from build123d import *

# Parameters (mm, degrees)
SKETCH1_W                   = 32.5
SKETCH1_H                   = 4.2
BASEFORM_DEPTH              = 7
SKETCH2_R                   = 0.75
HUMERUSAXLEHOLE1_DEPTH      = 2
HUMERUSAXLELOCK_DEPTH       = 1
SKETCH6_R                   = 1.5
AXLEEXTENSION_DEPTH         = 6
SKETCH7_R                   = 0.6
SCREWHOLES_DEPTH            = 54.273445543
SCREWHOLES_DEPTH_BACK       = 54.273445543
SKETCH8_W                   = 2.5
SKETCH8_H                   = 2.5
HUMERUSTUBEHOLDERBASE_DEPTH = 4.2
SKETCH13_W                  = 1.5
SKETCH13_H                  = 1.5
TUBECLIPENTRANCE_DEPTH      = 2
SKETCH14_W                  = 1.5
SKETCH14_H                  = 1.5
CABLECLIPLOCKSLOT_DEPTH     = 0.7
SKETCH15_W                  = 1.5
SKETCH15_H                  = 0.2
TUBECLIPLOCKCLEARANCE_DEPTH = 2
SKETCH12_R                  = 0.75
HUMERUSAXLEHOLE2_DEPTH      = 54.818584249


with BuildPart() as part:
    # Sketch1 → BaseForm (new body)
    with BuildSketch(Plane.XY):
        Polygon((0, -2.584500111), (0, 2.584500111), (3.25, 4.1), (39.25, 4.1), (42.5, 2.584500111), (42.5, -2.584500111), (39.25, -4.1), (3.25, -4.1), align=None)
        with Locations((21.25, 0)):
            Rectangle(SKETCH1_W, SKETCH1_H, mode=Mode.SUBTRACT)
    extrude(amount=BASEFORM_DEPTH)

    # Sketch2 → HumerusAxleHole1 (cut)
    with BuildSketch(Plane(origin=(0, 4.1, 0), x_dir=(1, 0, 0), z_dir=(0, 1, 0))):
        with Locations(Location((21.25, -3.5, 0), (0, 0, 270))):
            Circle(SKETCH2_R)
    extrude(amount=-HUMERUSAXLEHOLE1_DEPTH, mode=Mode.SUBTRACT)

    # Sketch2_4 → HumerusAxleLock (cut)
    with BuildSketch(Plane(origin=(0, 4.1, 0), x_dir=(1, 0, 0), z_dir=(0, 1, 0))):
        with BuildLine():
            ThreePointArc((20.65, -3.05), (21.25, -2.75), (21.85, -3.05))
            Line((21.85, -3.05), (21.85, -1.5))
            Line((21.85, -1.5), (20.65, -1.5))
            Line((20.65, -1.5), (20.65, -3.05))
        make_face()
        with BuildLine():
            Line((21.85, -5.5), (21.85, -3.95))
            ThreePointArc((21.85, -3.95), (21.25, -4.25), (20.65, -3.95))
            Line((20.65, -3.95), (20.65, -5.5))
            Line((20.65, -5.5), (21.85, -5.5))
        make_face()
    extrude(amount=-HUMERUSAXLELOCK_DEPTH, mode=Mode.SUBTRACT)

    # Sketch5 → Axle (revolve)
    with BuildSketch(Plane.XY.offset(3.5), mode=Mode.PRIVATE) as axle_sk:
        Polygon((53, 0), (53, 1.5), (46.5, 1.5), (44, 2.584500111), (42.5, 2.584500111), (42.5, 0), align=None)
    axle = revolve(axle_sk.sketch.rotate(Axis((42.5, 0, 3.5), (1, 0, 0)), 90), axis=Axis((42.5, 0, 3.5), (1, 0, 0)))

    # Axle2: Axle across plane
    add(axle.mirror(Plane.ZY.offset(-21.25)))

    # Sketch6 → AxleExtension (add)
    with BuildSketch(Plane.ZY.offset(10.5)):
        with Locations((3.5, 0)):
            Circle(SKETCH6_R)
    extrude(amount=AXLEEXTENSION_DEPTH)

    # Sketch7 → ScrewHoles (cut, two sides)
    with BuildSketch(Plane.XY.offset(3.5)) as screwholes_sk:
        with Locations((-9, 0)):
            Circle(SKETCH7_R)
        with Locations((-15, 0)):
            Circle(SKETCH7_R)
        with Locations((51.5, 0)):
            Circle(SKETCH7_R)
    extrude(amount=SCREWHOLES_DEPTH, mode=Mode.SUBTRACT)
    extrude(screwholes_sk.sketch, amount=-SCREWHOLES_DEPTH_BACK, mode=Mode.SUBTRACT)

    # Sketch8 → HumerusTubeHolderBase (add)
    with BuildSketch(Plane(origin=(0, 2.1, 0), x_dir=(1, 0, 0), z_dir=(0, 1, 0))):
        with Locations((14.1, -4.75)):
            Rectangle(SKETCH8_W, SKETCH8_H)
    humerustubeholderbase = extrude(amount=-HUMERUSTUBEHOLDERBASE_DEPTH)

    # Sketch13 → TubeClipEntrance (cut)
    with BuildSketch(Plane.XY.offset(6)):
        with Locations((14.1, 0.65)):
            Rectangle(SKETCH13_W, SKETCH13_H)
    tubeclipentrance = extrude(amount=-TUBECLIPENTRANCE_DEPTH, mode=Mode.SUBTRACT)

    # Sketch14 → CableClipLockSlot (cut)
    with BuildSketch(Plane.XZ.offset(-1.4)):
        with Locations((14.1, 4.75)):
            Rectangle(SKETCH14_W, SKETCH14_H)
    cablecliplockslot = extrude(amount=-CABLECLIPLOCKSLOT_DEPTH, mode=Mode.SUBTRACT)

    # Sketch15 → TubeClipLockClearance (cut)
    with BuildSketch(Plane.XY.offset(6)):
        with Locations((14.1, 1.5)):
            Rectangle(SKETCH15_W, SKETCH15_H)
    tubecliplockclearance = extrude(amount=-TUBECLIPLOCKCLEARANCE_DEPTH, mode=Mode.SUBTRACT)

    # Sketch12 → HumerusAxleHole2 (cut, through all)
    with BuildSketch(Plane(origin=(0, -2.1, 0), x_dir=(1, 0, 0), z_dir=(0, 1, 0))):
        with Locations(Location((21.25, -3.5, 0), (0, 0, 323.130102354))):
            Circle(SKETCH12_R)
    extrude(amount=-HUMERUSAXLEHOLE2_DEPTH, mode=Mode.SUBTRACT)

    # TubeClipSlot2: HumerusTubeHolderBase, TubeClipEntrance, CableClipLockSlot, TubeClipLockClearance across plane
    add(humerustubeholderbase.mirror(Plane(origin=(21.25, 0, 0), x_dir=(0, 0, 1), z_dir=(1, 0, 0))))
    add(tubeclipentrance.mirror(Plane(origin=(21.25, 0, 0), x_dir=(0, 0, 1), z_dir=(1, 0, 0))), mode=Mode.SUBTRACT)
    add(cablecliplockslot.mirror(Plane(origin=(21.25, 0, 0), x_dir=(0, 0, 1), z_dir=(1, 0, 0))), mode=Mode.SUBTRACT)
    add(tubecliplockclearance.mirror(Plane(origin=(21.25, 0, 0), x_dir=(0, 0, 1), z_dir=(1, 0, 0))), mode=Mode.SUBTRACT)


solid = part.part
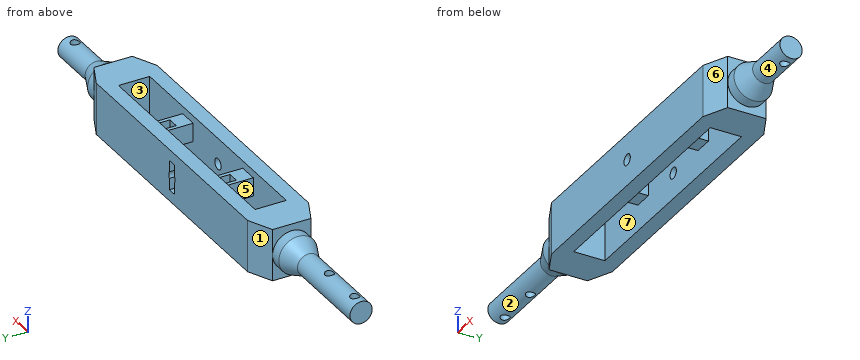
CAD build for the part. Positions are in the model's coordinates, mm. Face numbers are marked on the shaded views. A direction names the side the tool comes from. Round coordinates to 2 decimals unless told otherwise and drop trailing zeros. Write each loop counter-clockwise with the first axis right and the second up, starting at its lowest first coordinate (ties: lowest second). Pieces come first, ordered by that corner, then holes. Notation, with made-up numbers: M 70.25,21.25 L 107.25,21.25 A25 cw 107.25,50.25 Z; hole C 26,-18 d6. An arc over 180 degrees is marked long. Put each result on its own line as item: value. Start each with the question number.
1) 3-axis set-ups, long thin cutter, end or side, ignore diameter. For the marked faces 1, 2 and 3: which of +Z, -Z, +X, -X, +Y, -Y reach the whole face in a straight line?
2) Saw through at C-C, the plane x = 45. Write the cut outline in (y, z).
3) Saw through at A-A, the plane x = 10. Write the cut outline in (y, z).
4) Drill centre lines: probe 1 along X at (y, z) = (0, 2.9); probe 2 along Y at (x, z) = (28, 5.25); probe 3 along Z at (x, y) = (21.25, 2.6). Where is each one in solid material? Low to high. Write a range as [from, to].
5) Saw through at D-D, the plane x = -9. Write the cut outline in (y, z), and give its area (3 significant figures).
6) Pin check, flat tips, straight feed: pin 1 Ø0.8 at (x, y) = (28, 0.5) entering from +Z; pin 2 Ø0.8 at (y, z) = (3.5, 5) entering from -X; pin 3 Ø0.5 at (y, z) = (3.5, 2) entering from +X. Stop position of each tip, or through.
7) Saw through at B-B, the plane y = -3.25. Write the cut outline in (x, z).
8) Pull direction Y, two halves, no side cores. Call the marked faces 4, 5, 6 and 7: pulls with the +Y half, pulls with the -Y half, needs draft (parallel to the pull), parting line crosses it, or undercut.
Resolved:
1. face 1: +Z, -Z, -X, +Y
1. face 2: -X
1. face 3: +Z, -Z
2. outline: C 0,3.5 d4.3
3. outline: M -4.1,0 L -2.1,0 L -2.1,7 L -4.1,7 Z; M 2.1,0 L 4.1,0 L 4.1,7 L 2.1,7 Z
4. probe 1: [-16.5, -15.6], [-14.4, -9.6], [-8.4, 5], [37.5, 50.9], [52.1, 53]
4. probe 2: [-4.1, -0.1], [2.1, 4.1]
4. probe 3: [0, 2.75], [4.25, 7]
5. outline: M -0.6,2.13 L -0.6,4.87 A1.5 ccw Z; M 0.6,2.13 A1.5 ccw 0.6,4.87 Z
5. area: 3.57 mm²
6. pin 1: z = 6
6. pin 2: x = 1.11
6. pin 3: x = 41.07
7. outline: M 1.43,0 L 41.07,0 L 41.07,7 L 1.43,7 Z; hole C 21.25,3.5 d1.5
8. face 4: parting line crosses it
8. face 5: undercut
8. face 6: pulls with the -Y half
8. face 7: undercut
